Here's how the part is built. I have some questions about the finished solid (model axes, mm). A direction names the side the tool comes from. Give positions to 0.01 mm unless a question says otherwise; leave off trailing zeros. Loops run counter-clockwise (first coordinate to the right, second up) from the corner with the lowest first, then second, coordinate; pieces in that order, holes last.
Q1. Thinking about a two-plate mould opening in X: for faces 1 (the face through (-2.5, 9.1, 2.5)), 2 (the face through (3, 1.5, -0.3)), 3 (the face through (0.042, 4.393, -0.384)), 4 (the face through (0.24, 9.4, 2.65)), which applies, pulls with the +X half, pulls with the -X half, needs draft (parallel to the pull), parting line crosses it, or undercut?
Q2. Suppose I cut it at C-C (x = -1.35). List the corners of the cut face in (y, z) for me.
Q3. Suppose I cut it at D-D (x = 2.25). List the corners of the cut face in (y, z) for me, and give its area (3 significant figures).
Q4. Suppose I cut it at B-B (x = 0). List the corners of the cut face in (y, z) for me.
Q5. Suppose I cut it at A-A (y = 0). List the corners of the cut face in (x, z) for me.
Q6. I'm going to push flat-ended pins straight in: P1, Ø3, axis at x = 1, y = -1, coming from the +Z side; P2, Ø1, axis at x = 1.5, y = 9, coming from the -Z side; P3, Ø1, axis at x = -0.5, z = 2, coming from the +Y side. Where does each tip first touch, or does it pass through?
Q7. I need wall thicknesses on probe 1 along Z at (x, y) = (-1.25, 3.25); probe 2 along Y at (x, z) = (0, -0.15); probe 3 along X at (y, z) = (7.25, 1.45). Which ranges of each line are inside material? Lowest first, please.
Q8. For faces 5 (the face through (0, 2, -0.5)), 6 (the face through (0, 2, 0)), which set-ups out of +Z, -Z, +X, -X, +Y, -Y let a thin tool reach every point of the face, with its end or its side?
```python
from build123d import *

# Parameters (mm, degrees)
SKETCH_1_W             = 6
SKETCH_1_H             = 7
SM_BASE_FLANGE_1_DEPTH = 0.5
SM_EDGE_FLANGE_1_DEPTH = 6
SKETCH_11_R            = 1.5
CUT_EXTRUDE_1_DEPTH    = 14.480541017
CUT_EXTRUDE_2_REACH    = 15.287
SKETCH_12_R            = 0.8
OTHER_START            = 2.151923789
OTHER_1_DEPTH          = 0.5
OTHER_START_2          = -0.5
OTHER_1_2_DEPTH        = 0.5


# Read off the part's stored shape, not the designer's step: Затупленный угол1
# Sheet-metal steps are written as plain solids
with BuildPart() as part:
    # Sketch 1 → Базовая кромка1 (new body)
    with BuildSketch(Plane.XY):
        Rectangle(SKETCH_1_W, SKETCH_1_H)
    extrude(amount=-SM_BASE_FLANGE_1_DEPTH)

    # Ребро-кромка1 section (across the edge) → Ребро-кромка1 (add)
    with BuildSketch(Plane(origin=(3, 4.303847577, 0), x_dir=(0, -0.49999999999999495, 0.8660254037844416), z_dir=(-1, 0, 0))):
        with BuildLine():
            Line((-0.5, 0.803847577), (-0.5, 9))
            Line((-0.5, 9), (0, 9))
            Line((0, 9), (0, 0.803847577))
            ThreePointArc((0, 0.803847577), (0.102222521, 0.027390442), (0.401923789, -0.696152423))
            Line((0.401923789, -0.696152423), (-0.031088913, -0.946152423))
            ThreePointArc((-0.031088913, -0.946152423), (-0.380740392, -0.102019081), (-0.5, 0.803847577))
        make_face()
    extrude(amount=SM_EDGE_FLANGE_1_DEPTH)

    # Эскиз11 → Вырез-Вытянуть1 (cut, through all)
    with BuildSketch(Plane.XY):
        Circle(SKETCH_11_R)
    extrude(amount=-CUT_EXTRUDE_1_DEPTH, mode=Mode.SUBTRACT)

    # Эскиз12 → Вырез-Вытянуть2 (cut, up to next)
    with BuildSketch(Plane(origin=(0, 1.075961894, -1.863620668), x_dir=(1, 0, 0), z_dir=(0, -0.4999999999999949, 0.8660254037844416)), mode=Mode.PRIVATE) as cut_extrude_2_sk1:
        with Locations(Location((0, 10.227241336, 0), (0, 0, 270))):
            Circle(SKETCH_12_R)
    cut_extrude_2_tool1 = extrude(cut_extrude_2_sk1.sketch, amount=-CUT_EXTRUDE_2_REACH, mode=Mode.PRIVATE) & part.part
    # Эскиз12 → Вырез-Вытянуть2 (cut, up to next)
    with BuildSketch(Plane(origin=(0, 1.075961894, -1.863620668), x_dir=(1, 0, 0), z_dir=(0, -0.4999999999999949, 0.8660254037844416)), mode=Mode.PRIVATE) as cut_extrude_2_sk2:
        Polygon((-1.803847577, 12.727241336), (-2.5, 12.031088913), (-2.5, 6.227241336), (-3, 6.227241336), (-3, 12.727241336), align=None)
    cut_extrude_2_tool2 = extrude(cut_extrude_2_sk2.sketch, amount=-CUT_EXTRUDE_2_REACH, mode=Mode.PRIVATE) & part.part
    # Эскиз12 → Вырез-Вытянуть2 (cut, up to next)
    with BuildSketch(Plane(origin=(0, 1.075961894, -1.863620668), x_dir=(1, 0, 0), z_dir=(0, -0.4999999999999949, 0.8660254037844416)), mode=Mode.PRIVATE) as cut_extrude_2_sk3:
        Polygon((3, 12.727241336), (1.803847577, 12.727241336), (2.5, 12.031088913), (2.5, 6.227241336), (3, 6.227241336), align=None)
    cut_extrude_2_tool3 = extrude(cut_extrude_2_sk3.sketch, amount=-CUT_EXTRUDE_2_REACH, mode=Mode.PRIVATE) & part.part
    add(cut_extrude_2_tool1.solids().sort_by_distance((0, 9.933013, 3.25))[0], mode=Mode.SUBTRACT)
    add(cut_extrude_2_tool2.solids().sort_by_distance((-2.716553, 9.46484, 2.9797))[0], mode=Mode.SUBTRACT)
    add(cut_extrude_2_tool3.solids().sort_by_distance((2.716553, 9.46484, 2.9797))[0], mode=Mode.SUBTRACT)

    # Other 1 outline → Other 1 (cut)
    with BuildSketch(Plane(origin=(0, 0, 0), x_dir=(1, 0, 0), z_dir=(0, 0.4999999999999948, -0.8660254037844417)).offset(OTHER_START)):
        with BuildLine():
            Line((-3, -6.227241336), (-2.8, -6.227241336))
            ThreePointArc((-2.8, -6.227241336), (-2.941421356, -6.168662692), (-3, -6.027241336))
            Line((-3, -6.027241336), (-3, -6.227241336))
        make_face()
        with BuildLine():
            Line((-2.5, -12.031088913), (-2.441421356, -12.089667557))
            ThreePointArc((-2.441421356, -12.089667557), (-2.484775907, -12.024782888), (-2.5, -11.948246201))
            Line((-2.5, -11.948246201), (-2.5, -12.031088913))
        make_face()
        with BuildLine():
            Line((-1.803847577, -12.727241336), (-1.721004865, -12.727241336))
            ThreePointArc((-1.721004865, -12.727241336), (-1.797541551, -12.712017242), (-1.862426221, -12.668662692))
            Line((-1.862426221, -12.668662692), (-1.803847577, -12.727241336))
        make_face()
        with BuildLine():
            Line((1.803847577, -12.727241336), (1.862426221, -12.668662692))
            ThreePointArc((1.862426221, -12.668662692), (1.797541551, -12.712017242), (1.721004865, -12.727241336))
            Line((1.721004865, -12.727241336), (1.803847577, -12.727241336))
        make_face()
        with BuildLine():
            Line((2.5, -12.031088913), (2.5, -11.948246201))
            ThreePointArc((2.5, -11.948246201), (2.484775907, -12.024782888), (2.441421356, -12.089667557))
            Line((2.441421356, -12.089667557), (2.5, -12.031088913))
        make_face()
        with BuildLine():
            ThreePointArc((3, -6.027241336), (2.941421356, -6.168662692), (2.8, -6.227241336))
            Line((2.8, -6.227241336), (3, -6.227241336))
            Line((3, -6.227241336), (3, -6.027241336))
        make_face()
    extrude(amount=OTHER_1_DEPTH, mode=Mode.SUBTRACT)

    # Other 1 2 outline → Other 1 2 (cut)
    with BuildSketch(Plane.XY.offset(OTHER_START_2)):
        with BuildLine():
            ThreePointArc((3, -3.3), (2.941421356, -3.441421356), (2.8, -3.5))
            Line((2.8, -3.5), (3, -3.5))
            Line((3, -3.5), (3, -3.3))
        make_face()
        with BuildLine():
            ThreePointArc((-2.8, -3.5), (-2.941421356, -3.441421356), (-3, -3.3))
            Line((-3, -3.3), (-3, -3.5))
            Line((-3, -3.5), (-2.8, -3.5))
        make_face()
    extrude(amount=OTHER_1_2_DEPTH, mode=Mode.SUBTRACT)


solid = part.part
```
Solutions:
1. face 1: pulls with the -X half
1. face 2: pulls with the +X half
1. face 3: needs draft
1. face 4: undercut
2. outline: (-3.5, -0.5) - (-0.65, -0.5) - (-0.65, 0) - (-3.5, 0) - close; (0.65, -0.5) - (3.5, -0.5) arc R3.5 ccw to (5.25, -0.03) - (12.35, 4.07) - (12.1, 4.5) - (5, 0.4) arc R3 cw to (3.5, 0) - (0.65, 0) - close
3. outline: (-3.5, -0.5) - (3.5, -0.5) arc R3.5 ccw to (5.25, -0.03) - (11.96, 3.84) - (11.71, 4.28) - (5, 0.4) arc R3 cw to (3.5, 0) - (-3.5, 0) - close
3. area: 8.23 mm2
4. outline: (-3.5, -0.5) - (-1.5, -0.5) - (-1.5, 0) - (-3.5, 0) - close; (1.5, -0.5) - (3.5, -0.5) arc R3.5 ccw to (5.25, -0.03) - (9.49, 2.42) - (9.24, 2.85) - (5, 0.4) arc R3 cw to (3.5, 0) - (1.5, 0) - close; (10.63, 3.65) - (10.88, 3.22) - (12.35, 4.07) - (12.1, 4.5) - close
5. outline: (-3, -0.5) - (-1.5, -0.5) - (-1.5, 0) - (-3, 0) - close; (1.5, -0.5) - (3, -0.5) - (3, 0) - (1.5, 0) - close
6. P1: stops at z = 0
6. P2: stops at z = 1.85
6. P3: stops at y = 9.63
7. probe 1: z = -0.5 to 0
7. probe 2: y = -3.5 to -1.5, 1.5 to 5.03
7. probe 3: x = -2.5 to 2.5
8. face 5: -Z, +X, -X, +Y, -Y
8. face 6: +Z, +X, -X, -Y
